Verification items for the finished model (mm, model axes). Face numbers are marked on the shaded views. Round coordinates to 2 decimals unless told otherwise and drop trailing zeros. Order: outer loops, then holes, each group sorted by start corner. A loop starts at its lowest first (then second) coordinate and runs counter-clockwise, first axis right, second up. Notation, with made-up numbers: (74, -1) -> (118, -1) arc R3 ccw to (118, 4) -> close; hole circle Ø7 at (65.5, 12.25). An arc over 180 degrees is marked (long way). Put each result on its own line as item: value.
Autodesk Inventor part; units mm, degrees
ref_plane "YZ Plane" through (0, 0, 0) normal (1, 0, 0) x (0, 1, 0)
ref_plane "XZ Plane" through (0, 0, 0) normal (0, 1, 0) x (-1, 0, 0)
ref_plane "XY Plane" through (0, 0, 0) normal (0, 0, 1) x (1, 0, 0)
sketch "草图1" plane through (0, 0, 0) normal (0, 1, 0) x (-1, 0, 0)
  circle A0 centre (0, 0) radius 67.5
  dimension "d0" = 135
extrude "拉伸1" add sketch "草图1" along normal blind 17
sketch "草图3" plane through (0, 17, 0) normal (0, 1, 0) x (1, 0, 0)
  circle A0 centre (35, -35) radius 4
  point P0 (0, 0)
  dimension "d8" = 8
  dimension "d9" = 35
  dimension "d10" = 35
extrude "拉伸3" add sketch "草图3" along normal blind 1
shell "抽壳1" thickness 1.8 removed faces 1 at (33.7054, 18, 35.3191)
sketch "草图6" plane through (0, 17, 0) normal (0, 1, 0) x (1, 0, 0)
  circle A0 centre (0, 0) radius 36
  dimension "d17" = 72
extrude "拉伸5" cut sketch "草图6" against normal blind 1
sketch "草图7" plane through (0, 0, 0) normal (0, -1, 0) x (1, 0, 0)
  circle A0 centre (-12.941, 48.2963) radius 5
  line L0 (0, 0) -> (-12.941, 48.2963)
  line L1 (-94.5, 0) -> (94.5, 0)
  circle A1 centre (35, 35) radius 2.2
  line L2 (0, 0) -> (35, 35)
  dimension "d25" = 10
  dimension "d26" = 50
  dimension "d42" = 60
extrude "拉伸6" cut sketch "草图7" against normal blind 2 contours A0
pattern_circular "环形阵列1" count 3 over 360 about axis through (0, 17, 0) along (0, -1, 0) of "拉伸3"
sketch "草图8" plane through (12.8109, 18, -47.8109) normal (0, 1, 0) x (1, 0, 0)
  circle A0 centre (0, 0) radius 2
  point P0 (-12.8109, -47.8109)
  dimension "d32" = 4
extrude "拉伸7" cut sketch "草图8" against normal blind 3
sketch "草图9" plane through (-47.8109, 18, 12.8109) normal (0, 1, 0) x (1, 0, 0)
  circle A0 centre (0, 0) radius 2
  point P0 (47.8109, 12.8109)
  dimension "d35" = 4
extrude "拉伸8" cut sketch "草图9" against normal blind 3
pattern_circular "环形阵列2" count 3 over 360 about axis through (0, 0, 0) along (0, 1, 0) of "拉伸6"
properties part number "底盘" material "水"
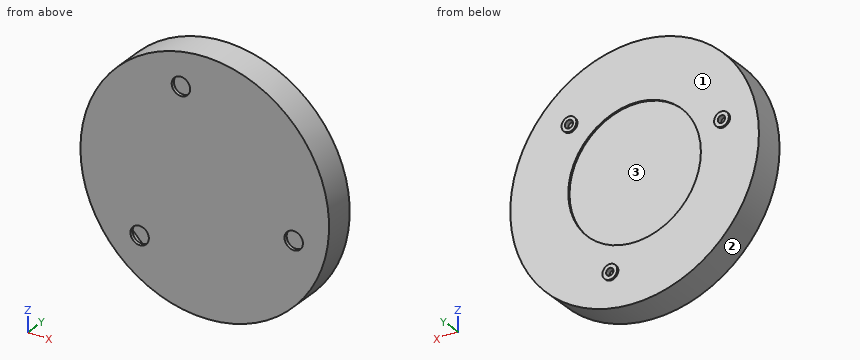
Item 1: Sectioned sample at B-B, the plane z = 0. Record the boundary of the cut face in (x, y), then the cut area to 3 significant figures.
Geometry check:
outline: (-67.5, 0) -> (67.5, 0) -> (67.5, 17) -> (36, 17) -> (36, 16) -> (-36, 16) -> (-36, 17) -> (-67.5, 17) -> close; hole (-65.7, 1.8) -> (65.7, 1.8) -> (65.7, 15.2) -> (-65.7, 15.2) -> close
area: 462 mm2
Item 2: Sectioned sample at D-D, the plane z = -58. Record the boundary of the cut face in (x, y).
Geometry check:
outline: (-34.53, 0) -> (34.53, 0) -> (34.53, 17) -> (-34.53, 17) -> close; hole (-30.86, 1.8) -> (30.86, 1.8) -> (30.86, 15.2) -> (-30.86, 15.2) -> close
Item 3: Depth check by flat-ended pin: pin 1 Ø1 at (x, y) = (7.5, 5) entering from +Z; pin 2 Ø11.5 at (x, z) = (48.3, -12.94) entering from -Y; pin 3 Ø2 at (x, y) = (-41, 7) entering from -Z; pin 4 Ø6 at (x, z) = (-12.94, 48.3) entering from +Y. Enter the tip coordinate at first touch or a pass-through.
Geometry check:
pin 1: z = 67.14
pin 2: y = 0
pin 3: z = -54.37
pin 4: y = 17
Item 4: Release check for a two-part mould opening along X. For the marked faces 1, 2 and 3 record: pulls with the +X half, pulls with the -X half, needs draft (parallel to the pull), parting line crosses it, or undercut.
Geometry check:
face 1: needs draft
face 2: parting line crosses it
face 3: undercut
Item 5: Sectioned sample at C-C, the plane y = 6. Record the boundary of the cut face in (x, z).
Geometry check:
outline: circle Ø135 at (0, 0); hole circle Ø131.4 at (0, 0)
Item 6: Material ranges on line 1 along Y through (x, z) = (20, 7.5); line 2 along Z through (x, y) = (1.5, 7); line 3 along Y through (x, z) = (-54.5, -24), recorded low to high.
Geometry check:
line 1: 0 to 1.8, 15.2 to 16
line 2: -67.48 to -65.68, 65.68 to 67.48
line 3: 0 to 1.8, 15.2 to 17
Item 7: Sectioned sample at A-A, the plane x = 0. Record the boundary of the cut face in (y, z).
Geometry check:
outline: (0, -67.5) -> (17, -67.5) -> (17, -36) -> (16, -36) -> (16, 36) -> (17, 36) -> (17, 67.5) -> (0, 67.5) -> close; hole (1.8, -65.7) -> (15.2, -65.7) -> (15.2, 65.7) -> (1.8, 65.7) -> close
